Here's the drawing with two shaded views (mm, measured from the low corner). I have some questions. Give positions to 0.01 mm unless a question says otherwise; leave off trailing zeros. Write each loop counter-clockwise with the first axis right and the second up, starting at its lowest first coordinate (ties: lowest second). Pieces come first, ordered by that corner, then holes. Notation, with made-up numbers: M -11.75,74 L -3.75,74 A15 cw -3.75,103 Z; hole C 27,64.25 d2. An arc over 180 degrees is marked long. Use one line per item in the form item = value. Start each with the question number.
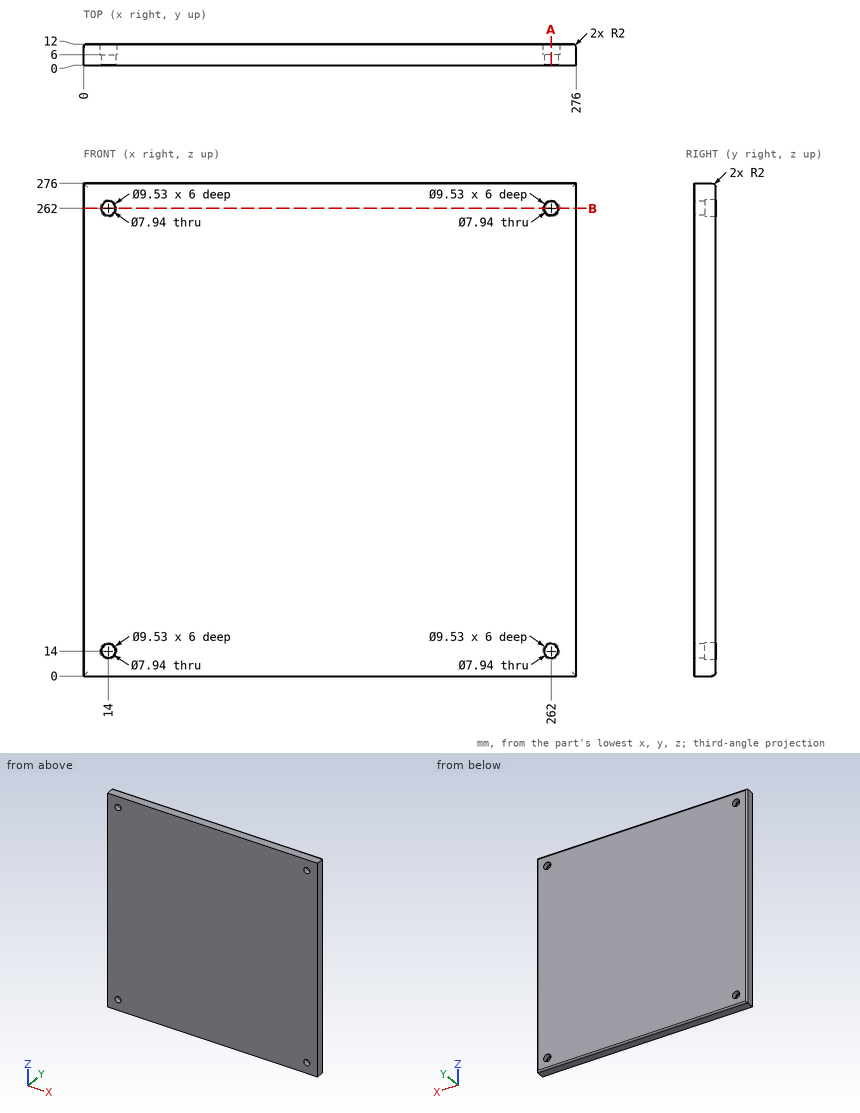
1) Suppose I cut it at B-B, the plane z = 262. List the corners of the cut face in (x, y) for me (3 decimals), and give its area (3 significant figures).
2) Please list where these lines run through material, in increasing order: line 1 (X direction, y = 2.85, z = 262); line 2 (Z direction, x = 262, y = 10.4) (3 decimals).
3) Will this pin go through, and if not, where does the flat tip stop? P1, Ø8.5, axis at x = 14, z = 262, coming from the +Y side.
4) Suppose I cut it at A-A, the plane x = 262. List the corners of the cut face in (y, z) for me (3 decimals).
Checks:
q1.outline = M 0,0 L 10.03,0 L 10.03,6 L 9.235,6 L 9.235,12 L 2,12 A2 ccw 0,10 Z; M 17.97,0 L 258.03,0 L 258.03,6 L 257.235,6 L 257.235,12 L 18.765,12 L 18.765,6 L 17.97,6 Z; M 265.97,0 L 276,0 L 276,10 A2 ccw 274,12 L 266.765,12 L 266.765,6 L 265.97,6 Z
q1.area = 3,100 mm^2
q2.line_1 = 0 to 10.03, 17.97 to 258.03, 265.97 to 276
q2.line_2 = 0.04 to 9.235, 18.765 to 257.235, 266.765 to 275.96
q3.P1 = 6
q4.outline = M 0,0 L 10,0 A2 ccw 12,2 L 12,9.235 L 6,9.235 L 6,10.03 L 0,10.03 Z; M 0,17.97 L 6,17.97 L 6,18.765 L 12,18.765 L 12,257.235 L 6,257.235 L 6,258.03 L 0,258.03 Z; M 0,265.97 L 6,265.97 L 6,266.765 L 12,266.765 L 12,274 A2 ccw 10,276 L 0,276 Z
